Part model, mm, in its own coordinate system. Coordinates: 2 decimals unless noted, no trailing zeros. Order: outer loops, then holes, each group sorted by start corner. A loop starts at its lowest first (then second) coordinate and runs counter-clockwise, first axis right, second up.
Autodesk Inventor part; units mm, degrees
ref_plane "Work Plane1" through (0, 0, 0) normal (0, 0, -1) x (-1, 0, 0)
ref_plane "YZ Plane" through (0, 0, 0) normal (1, 0, 0) x (0, 1, 0)
ref_plane "XZ Plane" through (0, 0, 0) normal (0, 1, 0) x (-1, 0, 0)
sketch "Sketch1" plane through (0, 0, 0) normal (0, 0, 1) x (1, 0, 0)
  circle A0 centre (-39.737, 23.1752) radius 3 construction
  circle A1 centre (-39.737, 23.1752) radius 19.05 construction
  circle A2 centre (-7.0783, -15.7355) radius 31.75 construction
  line L0 (-66.3054, -3.825) -> (-66.3054, -14.1122) construction
  line L1 (-66.3054, -14.1122) -> (-40.9054, -14.1122) construction
  line L2 (-40.9054, -14.1122) -> (-40.9054, -3.825) construction
  line L3 (-40.9054, -3.825) -> (-66.3054, -3.825) construction
  circle A3 centre (-7.0783, -15.7355) radius 3.81
  line L4 (-7.0783, -15.7355) -> (-33.4747, -30.9755) construction
  circle A4 centre (-18.0768, -22.0855) radius 2.3368
  circle A5 centre (-29.0753, -28.4355) radius 2.3368
  circle A6 centre (4.713, 16.8252) radius 9.525
  circle A7 centre (30.113, 16.8252) radius 9.525
  circle A8 centre (-29.0753, -28.4355) radius 9.525
  circle A9 centre (-7.0783, -15.7355) radius 9.525
  line L5 (-37.7116, -24.0819) -> (-2.9197, 22.5233)
  line L6 (-24.3128, -36.6844) -> (-2.3158, -23.9844)
  line L7 (-0.804, -22.9021) -> (36.3873, 9.6587)
  line L8 (4.713, 26.3502) -> (30.113, 26.3502)
  circle A10 centre (4.713, 16.8252) radius 2.3114
  circle A11 centre (30.113, 16.8252) radius 2.0828
  point P0 (0, 0)
  point P1 (-36.708, -22.7375)
  point P2 (4.713, 26.3502)
  dimension "d1" = 63.5
  dimension "d0" = 38.1
  dimension "d2" = 25.4
  dimension "d4" = 30.48
  dimension "d5" = 4.6736
  dimension "d6" = 4.6736
  dimension "d7" = 150
  dimension "d8" = 12.7
  dimension "d9" = 12.7
  dimension "d10" = 19.05
  dimension "d11" = 19.05
  dimension "d12" = 19.05
  dimension "d13" = 19.05
ref_plane "Work Plane1" through (0, 0, 0) normal (0, 0, -1) x (-1, 0, 0)
extrude "Extrusion2" add sketch "Sketch1" along normal blind 1.5875
sketch "Sketch3" plane through (0, 0, 0) normal (0, 0, -1) x (-1, 0, 0)
  circle A0 centre (7.0783, -15.7355) radius 3.81 construction
  circle A1 centre (7.0783, -15.7355) radius 32.8018 construction
  circle A2 centre (29.0753, -28.4355) radius 2.3368 construction
  circle A3 centre (29.0753, -28.4355) radius 2.3368 construction
  circle A4 centre (18.0768, -22.0855) radius 2.3368 construction
  circle A5 centre (18.0768, -22.0855) radius 2.3368 construction
  line L0 (18.0768, -22.0855) -> (29.0753, -28.4355) construction
  line L1 (29.0753, -28.4355) -> (40.0738, -34.7855) construction
  circle A6 centre (40.0738, -34.7855) radius 2.3368
  circle A7 centre (40.0738, -34.7855) radius 9.525
  circle A8 centre (-4.713, 16.8252) radius 2.3114
  circle A9 centre (-4.713, 16.8252) radius 9.525
  circle A10 centre (7.0783, -15.7355) radius 9.525
  line L2 (35.3113, -43.0344) -> (2.3158, -23.9844)
  line L3 (47.2678, -28.5428) -> (2.4809, 23.068)
  arc A11 (2.9197, 22.5233) -> (-4.713, 26.3502) centre (-4.713, 16.8252) ccw
  line L4 (-30.113, 26.3502) -> (-4.713, 26.3502)
  arc A12 (-30.113, 26.3502) -> (-36.3873, 9.6587) centre (-30.113, 16.8252) ccw
  line L5 (0.804, -22.9021) -> (-36.3873, 9.6587)
  arc A13 (0.804, -22.9021) -> (2.3158, -23.9844) centre (7.0783, -15.7355) ccw
  line L6 (24.3128, -36.6844) -> (2.3158, -23.9844)
  arc A14 (24.3128, -36.6844) -> (36.708, -22.7375) centre (29.0753, -28.4355) ccw
  line L7 (2.9197, 22.5233) -> (36.708, -22.7375)
  circle A15 centre (-30.113, 16.8252) radius 2.0828
  circle A16 centre (7.0783, -15.7355) radius 3.81
  circle A17 centre (29.0753, -28.4355) radius 2.3368
  circle A18 centre (-4.713, 16.8252) radius 2.3114
  circle A19 centre (18.0768, -22.0855) radius 2.3368
  point P0 (0, 0)
  point P1 (2.9197, 22.5233)
  dimension "d21" = 19.05
  dimension "d22" = 19.05
  dimension "d18" = 12.7
  dimension "d19" = 4.6736
  dimension "d20" = 19.05
extrude "Extrusion3" add sketch "Sketch3" against normal blind 1.5875 contours A7 A14 | A7 A14 L7 A9 L3 | L2 A14 A7 picked at (41.1437, -29.5718)
sketch "Sketch4" plane through (0, 0, 1.5875) normal (0, 0, 1) x (1, 0, 0)
  circle A0 centre (-29.0753, -28.4355) radius 2.3368
  circle A1 centre (-18.0768, -22.0855) radius 2.3368
  point P0 (0, 0)
extrude "Extrusion4" add sketch "Sketch4" against normal up to surface (1.5875 mm away)
properties part number "intakeMotor"
Q1. Cut at D-D on y = -4. Write the cut outline in (x, z).
Results list:
outline: (-25.97, 0) - (20.79, 0) - (20.79, 1.59) - (-25.97, 1.59) - close
Q2. Cut at A-A on x = -40.5. Write the cut outline in (y, z).
Results list:
outline: (-44.3, 0) - (-37.08, 0) - (-37.08, 1.59) - (-44.3, 1.59) - close; (-32.49, 0) - (-20.74, 0) - (-20.74, 1.59) - (-32.49, 1.59) - close
Q3. Cut at B-B on z = 0.7. Count the separate pieces of the cut face and the enclosed holes in it, and give its area (3 significant figures).
Results list:
separate pieces: 1
enclosed holes: 4
area: 2,760 mm2
Q4. Cut at C-C on x = -31. Write the cut outline in (y, z), and give its area (3 significant figures).
Results list:
outline: (-40.55, 0) - (-9.8, 0) - (-9.8, 1.59) - (-40.55, 1.59) - close
area: 48.8 mm2
Q5. Pin check, flat tips, straight feed: pin 1 Ø6 at (x, y) = (-7.08, -15.74) entering from -Z; pin 2 Ø6 at (x, y) = (4.71, 16.83) entering from +Z. Stop position of each tip, or through.
Results list:
pin 1: passes through
pin 2: stops at z = 1.59
Q6. Mould opens along X. For faces 1 (the face through (-5.32, -12.355, 0.783)), 2 (the face through (-19.04, -33.64, 0.78)), 3 (the face through (-6, -8, 0)) say: pulls with the +X half, pulls with the -X half, needs draft (parallel to the pull), parting line crosses it, or undercut.
Results list:
face 1: undercut
face 2: pulls with the +X half
face 3: needs draft
Q7. Wall check: line 1 along X through (y, z) = (-36.5, 1.35); line 2 along Y through (x, z) = (29, 0.4); line 3 along X through (y, z) = (-16, 1.3). Give the ranges that are in metal, low to high.
Results list:
line 1: x = -49.44 to -41.66, -38.49 to -23.99
line 2: y = 3.19 to 15.06, 18.59 to 26.35
line 3: x = -36.38 to -10.88, -3.28 to 7.08
